Read the model definition and answer for the solid it produces. Units are mm, in the model's axes. Face numbers are marked on the shaded views. A direction names the side the tool comes from. Round coordinates to 2 decimals unless told otherwise and drop trailing zeros. Order: outer loops, then holes, each group sorted by start corner. A loop starts at its lowest first (then second) coordinate and runs counter-clockwise, first axis right, second up. Notation, with made-up numbers: (74.25, -33.5) -> (99.25, -33.5) arc R12 cw to (99.25, -13.5) -> close; hole circle Ø11 at (57.25, 41). An arc over 180 degrees is marked (long way). Use a Markdown table: item, result. Add a question column.
1. Consider L1, parallel to Y at x = -14.5, z = -9; L2, parallel to Z at x = -11, y = -8.5; L3, parallel to X at y = -1.75, z = 32.5 (3 decimals). Determine where each line is inside the solid, lowest interval first. Write a range as [from, to].
2. Section C-C, the plane z = 8 is taken. Give the vertices of the cut face in (x, y).
3. Section A-A, the plane y = -4 is taken. Give the vertices of the cut face in (x, z), then the cut area to 3 significant figures.
4. Given pin 1 (4 mm diameter, centred on x = 17.5, z = 32.5, fed in from -Y); pin 2 (6 mm diameter, centred on x = 22, y = -2, fed in from +Z); pin 3 (3 mm diameter, centred on x = 5, z = 18.5, fed in from -Y), each flat-ended and moving along its own axis, determine where each tip first touches the part or whether it passes through.
5. Section B-B, the plane x = -6 is taken. Give the vertices of the cut face in (y, z), then the cut area to 3 significant figures.
6. Section D-D, the plane z = -17 is taken. Give the vertices of the cut face in (x, y).
7. For the marked faces 1, 2 and 3, determine the directions among +Z, -Z, +X, -X, +Y, -Y from which every point of the face is accessible in a straight line to the end or side of a thin tool.
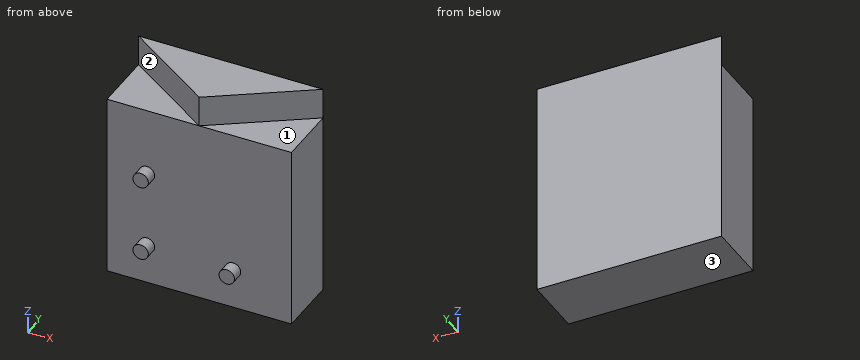
```python
from build123d import *

# Parameters (mm, degrees)
F0_W          = 20
F0_H          = 60
F1_DEPTH      = 30
F1_DEPTH_BACK = 30
F3_DEPTH      = 10
F4_R          = 2.5
F5_DEPTH      = 4


with BuildPart() as f1:
    # F0 (on Right) → F1 (new body, two sides)
    with BuildSketch(Plane.YZ) as f1_sk:
        Rectangle(F0_W, F0_H)
    extrude(amount=F1_DEPTH)
    extrude(f1_sk.sketch, amount=-F1_DEPTH_BACK)

    # F2 (on face) → F3 (join)
    with BuildSketch(Plane.XY.offset(30)):
        Polygon((30, 10), (-30, 10), (0, -10), align=None)
    extrude(amount=F3_DEPTH)

    # F4 (on face) → F5 (join)
    with BuildSketch(Plane.XZ.offset(10)):
        with Locations((-17, 8)):
            Circle(F4_R)
        with Locations((-17, -17)):
            Circle(F4_R)
        with Locations((11, -17)):
            Circle(F4_R)
    extrude(amount=F5_DEPTH)


solid = f1.part
```
Verdict:
| question | item | result |
|---|---|---|
| 1 | L1 | y = [-10, 10] |
| 1 | L2 | z = [-30, 30] |
| 1 | L3 | x = [-12.375, 12.375] |
| 2 | outline | (-30, -10) -> (-19.5, -10) -> (-19.5, -14) -> (-14.5, -14) -> (-14.5, -10) -> (30, -10) -> (30, 10) -> (-30, 10) -> close |
| 3 | outline | (-30, -30) -> (30, -30) -> (30, 30) -> (9, 30) -> (9, 40) -> (-9, 40) -> (-9, 30) -> (-30, 30) -> close |
| 3 | area | 3,780 mm2 |
| 4 | pin 1 | stops at y = 0.33 |
| 4 | pin 2 | stops at z = 30 |
| 4 | pin 3 | stops at y = -10 |
| 5 | outline | (-10, -30) -> (10, -30) -> (10, 40) -> (-6, 40) -> (-6, 30) -> (-10, 30) -> close |
| 5 | area | 1,360 mm2 |
| 6 | outline | (-30, -10) -> (-19.5, -10) -> (-19.5, -14) -> (-14.5, -14) -> (-14.5, -10) -> (8.5, -10) -> (8.5, -14) -> (13.5, -14) -> (13.5, -10) -> (30, -10) -> (30, 10) -> (-30, 10) -> close |
| 7 | face 1 | +Z, +X, -Y |
| 7 | face 2 | +Z, -X, -Y |
| 7 | face 3 | -Z, +X, -X, +Y, -Y |
